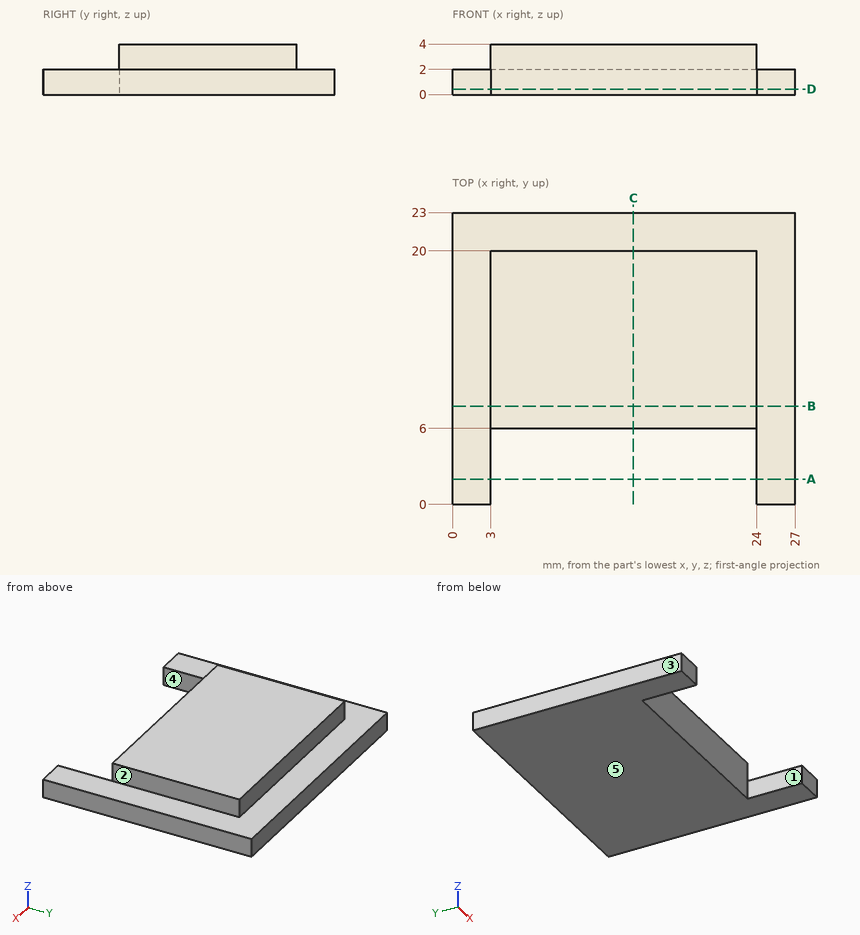
Could you check a few things on this drawing? It's one solid part, dimensions in mm from its lowest x, y, z. A direction names the side the tool comes from. Coordinates: 2 decimals unless noted, no trailing zeros. Order: outer loops, then holes, each group sorted by start corner. A loop starts at its lowest first (then second) coordinate and runs counter-clockwise, first axis right, second up. Notation, with made-up numbers: (35.25, 68.5) - (89.25, 68.5) arc R26 cw to (89.25, 101.5) - close; hole circle Ø1 at (64.25, -12). An arc over 180 degrees is marked (long way). Answer as a JSON object with one key per item and string values. Group by question number.
Q1. I need wall thicknesses on line 1 (X direction, y = 1.5, z = 1.3); line 2 (X direction, y = 10.5, z = 2.8); line 3 (Y direction, x = 16.5, z = 3.4). Which ranges of each line are inside material? Lowest first, please. Write a range as from..to.
Q2. Imagine slicing it at A-A (y = 2). Please give me the cut outline in (x, z).
Q3. Imagine slicing it at D-D (z = 0.45). Please give me the cut outline in (x, y), and give its area (3 significant figures).
Q4. We'd pull the mould along X, two halves only. Please class the marked faces 1, 2 and 3: +X half, -X half, draft (parallel to the pull), parting line (faces both ways), or undercut.
Q5. Will these pins go through, and if not, where does the flat tip stop? P1, Ø0.6, axis at y = 13.5, z = 3, coming from the +X side; P2, Ø0.6, axis at x = 17.5, z = 3, coming from the +Y side; P3, Ø1.6, axis at y = 12.5, z = 3, coming from the -X side.
Q6. Imagine slicing it at C-C (x = 14.25). Please give me the cut outline in (y, z), and give its area (3 significant figures).
Q7. Imagine slicing it at B-B (y = 7.75). Please give me the cut outline in (x, z).
Q8. On a 3-axis mill with a long thin cutter (end or side, diameter ignored), from which of +Z, -Z, +X, -X, +Y, -Y can I reach the whole of each face in a straight line? I mean the marked faces 4 and 5. Say none if no direction works.
Determined:
{
 "1": {"line 1": "x = 0..3, 24..27", "line 2": "x = 3..24", "line 3": "y = 6..20"},
 "2": {"outline": "(0, 0) - (3, 0) - (3, 2) - (0, 2) - close; (24, 0) - (27, 0) - (27, 2) - (24, 2) - close"},
 "3": {"outline": "(0, 0) - (3, 0) - (3, 6) - (24, 6) - (24, 0) - (27, 0) - (27, 23) - (0, 23) - close", "area": "495 mm2"},
 "4": {"face 1": "undercut", "face 2": "+X half", "face 3": "-X half"},
 "5": {"P1": "stops at x = 24", "P2": "stops at y = 20", "P3": "stops at x = 3"},
 "6": {"outline": "(6, 0) - (23, 0) - (23, 2) - (20, 2) - (20, 4) - (6, 4) - close", "area": "62.0 mm2"},
 "7": {"outline": "(0, 0) - (27, 0) - (27, 2) - (24, 2) - (24, 4) - (3, 4) - (3, 2) - (0, 2) - close"},
 "8": {"face 4": "+Z, -Z, -Y", "face 5": "-Z, +X, -X, +Y, -Y"}
}
